Source: CAD feature listing. Evaluate the final solid. Frame: model axes, mm. Face numbers are marked on the shaded views. A direction names the side the tool comes from. Give positions to 0.01 mm unless a question says otherwise; leave off trailing zeros. Write each loop counter-clockwise with the first axis right and the second up, starting at its lowest first coordinate (ties: lowest second). Pieces come first, ordered by that corner, then holes.
```python
from build123d import *

# Parameters (mm, degrees)
SKETCH_1_W          = 25
SKETCH_1_H          = 31
EXTRUDE_1_DEPTH     = 2
SKETCH_2_W          = 21
SKETCH_2_H          = 25
EXTRUDE_2_DEPTH     = 16
EXTRUDE_3_DEPTH     = 9.25
EXTRUDE_5_DEPTH     = 8.5
SKETCH_5_W          = 1
SKETCH_5_H          = 23
SKETCH_5_W_2        = 9
SKETCH_5_H_2        = 0.5
EXTRUDE_6_DEPTH     = 10
SKETCH_6_R          = 1.5
SKETCH_6_R_2        = 0.75
CUT_EXTRUDE_1_DEPTH = 27.688922773


with BuildPart() as part:
    # Эскиз1 → Бобышка-Вытянуть1 (new body)
    with BuildSketch(Plane(origin=(0, 0, 0), x_dir=(1, 0, 0), z_dir=(0, 1, 0))):
        Rectangle(SKETCH_1_W, SKETCH_1_H)
    extrude(amount=EXTRUDE_1_DEPTH)

    # Эскиз2 → Бобышка-Вытянуть2 (add)
    with BuildSketch(Plane.XZ):
        Rectangle(SKETCH_2_W, SKETCH_2_H)
    extrude(amount=EXTRUDE_2_DEPTH)

    # Эскиз3 → Бобышка-Вытянуть3 (add, symmetric)
    with BuildSketch(Plane(origin=(0, 0, 0), x_dir=(0, 0, -1), z_dir=(1, 0, 0))):
        with BuildLine():
            Line((11, 2), (-11, 2))
            Line((-11, 2), (-10, 6))
            ThreePointArc((-10, 6), (0, 5), (10, 6))
            Line((10, 6), (11, 2))
        make_face()
    extrude(amount=EXTRUDE_3_DEPTH, both=True)

    # Эскиз4 → Бобышка-Вытянуть5 (add, symmetric)
    with BuildSketch(Plane(origin=(0, 0, 0), x_dir=(0, 0, -1), z_dir=(1, 0, 0))):
        Polygon((-12.5, -16), (-15.688922773, -3.397191918), (-13.42429798, -0.1), (-12.6, -0.666156198), (-14.608505885, -3.590450497), (-11.530553224, -15.754698248), align=None)
        Polygon((14.608505885, -3.590450497), (11.530553224, -15.754698248), (12.5, -16), (15.688922773, -3.397191918), (13.42429798, -0.1), (12.6, -0.666156198), align=None)
    extrude(amount=EXTRUDE_5_DEPTH, both=True)

    # Эскиз5 → Бобышка-Вытянуть6 (add)
    with BuildSketch(Plane.XZ.offset(16)):
        Rectangle(SKETCH_5_W, SKETCH_5_H)
        with Locations((5.5, -10.75)):
            Rectangle(SKETCH_5_W_2, SKETCH_5_H_2)
        with Locations((5.5, 10.75)):
            Rectangle(SKETCH_5_W_2, SKETCH_5_H_2)
        with Locations((5.5, 0)):
            Rectangle(SKETCH_5_W_2, SKETCH_5_H_2)
        with Locations((-5.5, -10.75)):
            Rectangle(SKETCH_5_W_2, SKETCH_5_H_2)
        with Locations((-5.5, 0)):
            Rectangle(SKETCH_5_W_2, SKETCH_5_H_2)
        with Locations((-5.5, 10.75)):
            Rectangle(SKETCH_5_W_2, SKETCH_5_H_2)
    extrude(amount=EXTRUDE_6_DEPTH)

    # Эскиз6 → Вырез-Вытянуть1 (cut, through all)
    with BuildSketch(Plane(origin=(0, 0, -11), x_dir=(-1, 0, 0), z_dir=(0, 0, -1))):
        with Locations((-5.5, -21.5)):
            Circle(SKETCH_6_R)
        with Locations((-5.5, -17.25)):
            Circle(SKETCH_6_R_2)
        with Locations((5.5, -17.25)):
            Circle(SKETCH_6_R_2)
        with Locations((5.5, -21.5)):
            Circle(SKETCH_6_R)
        Polygon((-10.25, -16.5), (-9, -16.5), (-9, -24), (-8, -26), (-8, -27.807511946), (-10.25, -27.807511946), align=None)
        Polygon((-3, -27.807511946), (-0.75, -27.807511946), (-0.75, -16.5), (-2, -16.5), (-2, -24), (-3, -26), align=None)
        Polygon((3, -26), (3, -27.807511946), (0.75, -27.807511946), (0.75, -16.5), (2, -16.5), (2, -24), align=None)
        Polygon((8, -27.807511946), (10.25, -27.807511946), (10.25, -16.5), (9, -16.5), (9, -24), (8, -26), align=None)
    extrude(amount=-CUT_EXTRUDE_1_DEPTH, mode=Mode.SUBTRACT)


solid = part.part
```
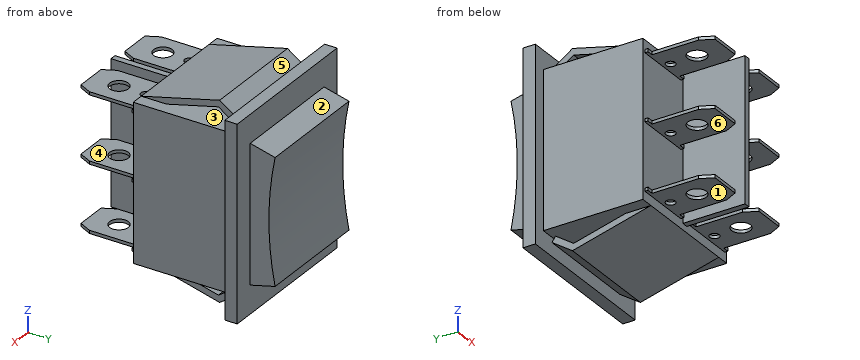
1. Line query: probe 1 along Y at (x, z) = (-5.5, -0.05); probe 2 along Z at (x, y) = (6.5, -24); probe 3 along Z at (x, y) = (1.25, -1). Output: solid intervals per line, ascending.
2. Pull-direction query (Y, two-part tool) for the marked faces 1, 2 and 3; classes: pulls with the +Y half, pulls with the -Y half, needs draft (parallel to the pull), parting line crosses it, or undercut.
3. Pin query (flat end, axial travel): P1, Ø10, axis at y = -15.5, z = 1.5, coming from the -X side; P2, Ø7, axis at x = -6.5, y = -22, coming from the -Z side; P3, Ø1.5, axis at x = 0.5, y = 0, coming from the +Z side. Return the tip coordinate at first contact, or that it passes through.
4. Access query for the marked faces 4, 5 and 6. Directions: +Z, -Z, +X, -X, +Y, -Y. A direction counts if a zero-diameter tool reaches every point of the face in a straight line with its end or side. Return the directions, or none.
5. Section query B-B (y = -17.25). Give the number of separate pieces and of enclosed holes in the cut face, plus the area to 3 significant figures.
6. Section query D-D (z = -8). Return loops of the section in (x, y).
The answers:
1. probe 1: y = -26 to -23, -20 to -18, -16.5 to 5
1. probe 2: z = -11 to -10.5, -0.25 to 0.25, 10.5 to 11
1. probe 3: z = -14.04 to -12.83, -12.5 to 12.5, 12.83 to 14.04
2. face 1: needs draft
2. face 2: pulls with the +Y half
2. face 3: undercut
3. P1: stops at x = -10.5
3. P2: stops at z = -11
3. P3: stops at z = 15.5
4. face 4: +X, -Y
4. face 5: +Z, +X, -X
4. face 6: -X, -Y
5. separate pieces: 13
5. enclosed holes: 0
5. area: 39.5 mm2
6. outline: (-12.5, 0) - (-10.5, 0) - (-10.5, -16) - (-0.5, -16) - (-0.5, -26) - (0.5, -26) - (0.5, -16) - (10.5, -16) - (10.5, 0) - (12.5, 0) - (12.5, 2) - (9.25, 2) - (9.25, 5.64) - (-9.25, 5.64) - (-9.25, 2) - (-12.5, 2) - close
